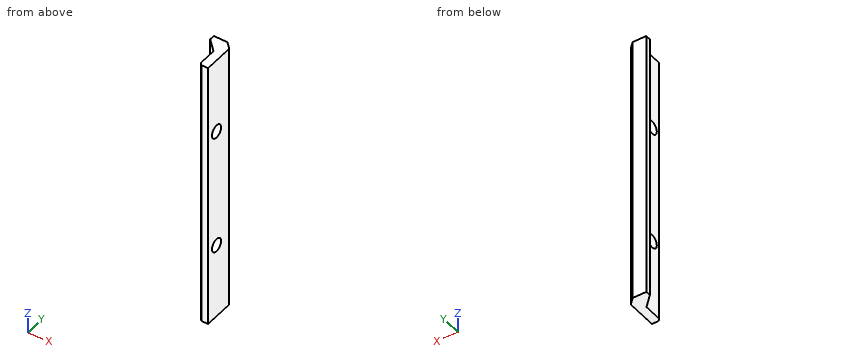
```python
from build123d import *

# Parameters (mm, degrees)
BOSS_EXTRUDE1_DEPTH = 90
CUT_EXTRUDE1_REACH  = 93.029
SKETCH4_R           = 2.15
FILLET1_R           = 1


with BuildPart() as part:
    # Sketch3 → Boss-Extrude1 (new body)
    with BuildSketch(Plane.XY):
        Polygon((3.617157288, -12), (3.617157288, -5.297157288), (0, -1.68), (0, 0), (4.5, 0), (6.5, -2), (6.5, -12), align=None)
    extrude(amount=BOSS_EXTRUDE1_DEPTH)

    # Sketch4 → Cut-Extrude1 (cut, up to next)
    with BuildSketch(Plane(origin=(6.5, 0, 0), x_dir=(0, 0, -1), z_dir=(1, 0, 0)), mode=Mode.PRIVATE) as cut_extrude1_sk1:
        with Locations((-65, -8)):
            Circle(SKETCH4_R)
    cut_extrude1_tool1 = extrude(cut_extrude1_sk1.sketch, amount=-CUT_EXTRUDE1_REACH, mode=Mode.PRIVATE) & part.part
    # Sketch4 → Cut-Extrude1 (cut, up to next)
    with BuildSketch(Plane(origin=(6.5, 0, 0), x_dir=(0, 0, -1), z_dir=(1, 0, 0)), mode=Mode.PRIVATE) as cut_extrude1_sk2:
        with Locations((-25, -8)):
            Circle(SKETCH4_R)
    cut_extrude1_tool2 = extrude(cut_extrude1_sk2.sketch, amount=-CUT_EXTRUDE1_REACH, mode=Mode.PRIVATE) & part.part
    add(cut_extrude1_tool1.solids().sort_by_distance((6.5, -8, 65))[0], mode=Mode.SUBTRACT)
    add(cut_extrude1_tool2.solids().sort_by_distance((6.5, -8, 25))[0], mode=Mode.SUBTRACT)

    # Fillet1
    fillet1_edges = [part.edges().sort_by_distance(p)[0] for p in [
        (3.617157288, -12, 45),
    ]]
    fillet(fillet1_edges, radius=FILLET1_R)


solid = part.part
```
The model under review builds one solid part; all positions refer to its coordinate system, in mm. Give positions to 0.01 mm unless a question says otherwise; leave off trailing zeros. Write each loop counter-clockwise with the first axis right and the second up, starting at its lowest first coordinate (ties: lowest second). Pieces come first, ordered by that corner, then holes. Notation, with made-up numbers: M -15,-35 L 23,-35 A10 ccw 23,-16 Z; hole C 16,53.5 d1. An arc over 180 degrees is marked long. Write each question's results on one line, items separated by ' | '. Start each with the question number.
1. Insertion check: pin 1 Ø1 at (x, y) = (3, -7) entering from -Z; pin 2 Ø3 at (y, z) = (-7.5, 25.5) entering from -X. Each pin has a flat end and moves straight along its axis. Give the tip position at first contact, or say it passes through.
2. We need section A-A (z = 25). Write out the cut boundary in (x, y), and give its area (3 significant figures).
3. We need section D-D (x = 2.5). Write out the cut boundary in (y, z).
4. We need section C-C (z = 40.5). Write out the cut boundary in (x, y).
5. For probe 1 along Z at (x, y) = (5, -6.5); probe 2 along X at (y, z) = (-7.5, 43); probe 3 along Y at (x, z) = (4.55, 65), list the stretches that pass through material, from the lowest coordinate up. Write a range as [from, to].
6. We need section B-B (y = -8). Write out the cut boundary in (x, z).
Results found:
1) pin 1: passes through | pin 2: stops at x = 3.62
2) outline: M 0,-1.68 L 3.62,-5.3 L 3.62,-5.85 L 6.5,-5.85 L 6.5,-2 L 4.5,0 L 0,0 Z; M 3.62,-11 A1 ccw 4.62,-12 L 6.5,-12 L 6.5,-10.15 L 3.62,-10.15 Z | area: 32.6 mm^2
3) outline: M -4.18,0 L 0,0 L 0,90 L -4.18,90 Z
4) outline: M 0,-1.68 L 3.62,-5.3 L 3.62,-11 A1 ccw 4.62,-12 L 6.5,-12 L 6.5,-2 L 4.5,0 L 0,0 Z
5) probe 1: z = [0, 23.46], [26.54, 63.46], [66.54, 90] | probe 2: x = [3.62, 6.5] | probe 3: y = [-12, -10.15], [-5.85, -0.05]
6) outline: M 3.62,0 L 6.5,0 L 6.5,22.85 L 3.62,22.85 Z; M 3.62,27.15 L 6.5,27.15 L 6.5,62.85 L 3.62,62.85 Z; M 3.62,67.15 L 6.5,67.15 L 6.5,90 L 3.62,90 Z
